```python
from build123d import *

# Parameters (mm, degrees)
SKETCH1_R           = 4
BOSS_EXTRUDE1_DEPTH = 3
SKETCH2_W           = 11
SKETCH2_H           = 1
CUT_EXTRUDE1_DEPTH  = 13.4


with BuildPart() as part:
    # Sketch1 → Boss-Extrude1 (new body)
    with BuildSketch(Plane(origin=(0, 0, 0), x_dir=(1, 0, 0), z_dir=(0, 1, 0))):
        Polygon((43, 7.7), (43, -7.7), (6, -7.7), (6, -26.7), (5.499093619, -27.3), (4.500906381, -27.3), (4, -26.7), (3.499093619, -27.3), (2.500906381, -27.3), (2, -26.7), (1.499093619, -27.3), (0.500906381, -27.3), (0, -26.7), (0, 7.7), align=None)
        with Locations(Location((16.5, 0, 0), (0, 0, 270))):
            Circle(SKETCH1_R, mode=Mode.SUBTRACT)
        with Locations(Location((28.5, 0, 0), (0, 0, 270))):
            Circle(SKETCH1_R, mode=Mode.SUBTRACT)
    extrude(amount=BOSS_EXTRUDE1_DEPTH)

    # Sketch2 → Cut-Extrude1 (cut)
    with BuildSketch(Plane.XY.offset(7.7)):
        with Locations((16.5, 1.5)):
            Rectangle(SKETCH2_W, SKETCH2_H)
        with Locations((28.5, 1.5)):
            Rectangle(SKETCH2_W, SKETCH2_H)
    extrude(amount=-CUT_EXTRUDE1_DEPTH, mode=Mode.SUBTRACT)


solid = part.part
```
Input: part model. Units: mm. Frame: model coordinates. A direction names the side the tool comes from. Round coordinates to 2 decimals unless told otherwise and drop trailing zeros. Order: outer loops, then holes, each group sorted by start corner. A loop starts at its lowest first (then second) coordinate and runs counter-clockwise, first axis right, second up. Notation, with made-up numbers: (-13, 10.5) - (44, 10.5) arc R18 ccw to (44, 28.5) - close; hole circle Ø9 at (48.25, 51.5). An arc over 180 degrees is marked (long way). Answer in a Markdown table with one row per item.
Item 1: Section query C-C (x = 28.5). Return the cut outline in (y, z).
Model answer:
| item | result |
|---|---|
| outline | (0, -7.7) - (3, -7.7) - (3, -4) - (2, -4) - (2, -5.7) - (1, -5.7) - (1, -4) - (0, -4) - close; (0, 4) - (1, 4) - (1, 7.7) - (0, 7.7) - close; (2, 4) - (3, 4) - (3, 7.7) - (2, 7.7) - close |
Item 2: Pin query (flat end, axial travel): pin 1 (12 mm diameter, centred on x = 19, z = 10.5, fed in from -Y); pin 2 (1.1 mm diameter, centred on x = 17, y = 1.5, fed in from +Z). Return the tip coordinate at first contact, or that it passes through.
Model answer:
| item | result |
|---|---|
| pin 1 | stops at y = 0 |
| pin 2 | stops at z = 7.7 |
Item 3: Section query A-A (z = 0). Return the cut outline in (x, y), then the cut area to 3 significant figures.
Model answer:
| item | result |
|---|---|
| outline | (0, 0) - (12.5, 0) - (12.5, 1) - (11, 1) - (11, 2) - (12.5, 2) - (12.5, 3) - (0, 3) - close; (20.5, 0) - (24.5, 0) - (24.5, 1) - (23, 1) - (23, 2) - (24.5, 2) - (24.5, 3) - (20.5, 3) - (20.5, 2) - (22, 2) - (22, 1) - (20.5, 1) - close; (32.5, 0) - (43, 0) - (43, 3) - (32.5, 3) - (32.5, 2) - (34, 2) - (34, 1) - (32.5, 1) - close |
| area | 75.0 mm² |
Item 4: Line query: line 1 (X direction, y = 1.65, z = -2); line 2 (X direction, y = 2.35, z = 0); line 3 (Z direction, x = 16.5, y = 2.45). Output: solid intervals per line, ascending.
Model answer:
| item | result |
|---|---|
| line 1 | x = 0 to 11, 22 to 23, 34 to 43 |
| line 2 | x = 0 to 12.5, 20.5 to 24.5, 32.5 to 43 |
| line 3 | z = -7.7 to -4, 4 to 7.7 |
Item 5: Reachability of faces 4 (the cylindrical face through (32.466, 0.493, -0.521)), 5 (the flat face through (28.4, 1.5, -5.7)) from +Z, -Z, +X, -X, +Y, -Y: full face, straight path, thin tool, end or side. Return the list, or none.
Model answer:
| item | result |
|---|---|
| face 4 | +Y, -Y |
| face 5 | +Z |
Item 6: Section query B-B (y = 2.55). Return the cut outline in (x, z).
Model answer:
| item | result |
|---|---|
| outline | (0, -7.7) - (43, -7.7) - (43, 7.7) - (6, 7.7) - (6, 26.7) - (5.5, 27.3) - (4.5, 27.3) - (4, 26.7) - (3.5, 27.3) - (2.5, 27.3) - (2, 26.7) - (1.5, 27.3) - (0.5, 27.3) - (0, 26.7) - close; hole circle Ø8 at (16.5, 0); hole circle Ø8 at (28.5, 0) |
Item 7: Section query D-D (z = 5.5). Return the cut outline in (x, y).
Model answer:
| item | result |
|---|---|
| outline | (0, 0) - (43, 0) - (43, 3) - (0, 3) - close; hole (11, 1) - (22, 1) - (22, 2) - (11, 2) - close; hole (23, 1) - (34, 1) - (34, 2) - (23, 2) - close |
Item 8: Mould query, pull axis Z, two halves, no side actions, for faces 1 (the flat face through (16.4, 1.5, -5.7)), 2 (the cylindrical face through (20.466, 0.493, -0.521)), 3 (the flat face through (11, 1.5, 1.1)). Classes: released by +Z, released by -Z, zero draft, split by the parting line, or undercut.
Model answer:
| item | result |
|---|---|
| face 1 | released by +Z |
| face 2 | undercut |
| face 3 | zero draft |
